Build history of the part. All positions in model axes, mm. A direction names the side the tool comes from. Coordinates: 2 decimals unless noted, no trailing zeros. Order: outer loops, then holes, each group sorted by start corner. A loop starts at its lowest first (then second) coordinate and runs counter-clockwise, first axis right, second up. Notation, with made-up numbers: (-19, 59) - (-13, 59) arc R20 ccw to (-13, 84) - close; hole circle Ø7 at (44.25, 82.25). An arc over 180 degrees is marked (long way). Write each question's results on one line, items separated by ' | '.
Autodesk Inventor part; units mm, degrees
ref_plane "Start plane" through (0, 0, -20) normal (0, 0, 1) x (1, 0, 0)
ref_plane "End plane" through (0, 0, 520) normal (0, 0, 1) x (1, 0, 0)
ref_plane "Work Plane4" through (20, 0, 520) normal (-0.7071, 0, 0.7071) x (0.7071, 0, 0.7071)
ref_plane "Start plane" through (0, 0, -20) normal (0, 0, 1) x (1, 0, 0)
ref_plane "End plane" through (0, 0, 520) normal (0, 0, 1) x (1, 0, 0)
sketch "Sketch" plane through (0, 0, 0) normal (0, 0, 1) x (1, 0, 0)
  line L0 (-20, -16.1) -> (-20, 16.1)
  line L1 (-16.1, 20) -> (16.1, 20)
  line L2 (20, 16.1) -> (20, -16.1)
  line L3 (16.1, -20) -> (-16.1, -20)
  arc A0 (-20, -16.1) -> (-16.1, -20) centre (-16.1, -16.1) ccw
  arc A1 (-16.1, 20) -> (-20, 16.1) centre (-16.1, 16.1) ccw
  arc A2 (20, 16.1) -> (16.1, 20) centre (16.1, 16.1) ccw
  arc A3 (16.1, -20) -> (20, -16.1) centre (16.1, -16.1) ccw
  line L4 (-14.8, 17.4) -> (14.8, 17.4)
  line L5 (17.4, 14.8) -> (17.4, -14.8)
  line L6 (14.8, -17.4) -> (-14.8, -17.4)
  line L7 (-17.4, -14.8) -> (-17.4, 14.8)
  line L8 (0, 29.1308) -> (0, -29.1308) construction
  line L9 (-29.1308, 0) -> (29.1308, 0) construction
  arc A4 (-17.4, -14.8) -> (-14.8, -17.4) centre (-14.8, -14.8) ccw
  arc A5 (-14.8, 17.4) -> (-17.4, 14.8) centre (-14.8, 14.8) ccw
  arc A6 (17.4, 14.8) -> (14.8, 17.4) centre (14.8, 14.8) ccw
  arc A7 (14.8, -17.4) -> (17.4, -14.8) centre (14.8, -14.8) ccw
  dimension "d7" = 3.9
  dimension "d10" = 40
  dimension "d11" = 40
  dimension "d12" = 2.6
  dimension "d15" = 20
  dimension "d16" = 20
  dimension "d19" = 2.6
  dimension "d20" = 2.6
extrude "Body" add sketch "Sketch" along normal up to surface (540 mm away) from surface at -20
sketch "Sketch3" plane through (0, 0, 0) normal (0, 0, 1) x (1, 0, 0)
  line L0 (0, 0) -> (10, 0)
ref_plane "Work Plane3" through (0, 0, 0) normal (0, -1, 0) x (1, 0, 0)
sketch "Sketch4" plane through (0, 0, 0) normal (0, -1, 0) x (1, 0, 0)
  line L0 (-2, -20) -> (12, -20)
  line L1 (-2, 520) -> (12, 520)
  dimension "d18" = 540
ref_plane "Work Plane4" through (20, 0, 520) normal (-0.7071, 0, 0.7071) x (0.7071, 0, 0.7071)
split "Split1" plane through (20, 0, 520) removes the side toward (-0.7071, 0, 0.7071)
ref_plane "Work Plane5" through (20, 0, -20) normal (-0.7071, 0, -0.7071) x (-0.7071, 0, 0.7071)
split "Split2" plane through (20, 0, -20) removes the side toward (-0.7071, 0, -0.7071)
equation "\"d7\" = G_IR"
equation "\"d10\" = G_H"
equation "\"d11\" = G_W"
equation "\"d12\" = G_T"
equation "\"d15\" = 0.5 * d10"
equation "\"d16\" = 0.5 * d11"
equation "\"d19\" = G_T"
equation "\"d20\" = G_T"
equation "\"d3\" = G_L"
equation "\"G_W\" = 40"
equation "\"G_H\" = 40"
equation "\"G_T\" = 2.6"
equation "\"G_IR\" = 3.9"
equation "\"G_L\" = d18"
properties part number "EN 10210-2 - 40 x 40 x 2.6 - 540" material "Steel, Galvanized"
1. Band-saw the part on C-C on z = 337.5. Give the cut face in (x, y).
Solved:
outline: (-20, -16.1) arc R3.9 ccw to (-16.1, -20) - (16.1, -20) arc R3.9 ccw to (20, -16.1) - (20, 16.1) arc R3.9 ccw to (16.1, 20) - (-16.1, 20) arc R3.9 ccw to (-20, 16.1) - close; hole (-17.4, -14.8) arc R2.6 ccw to (-14.8, -17.4) - (14.8, -17.4) arc R2.6 ccw to (17.4, -14.8) - (17.4, 14.8) arc R2.6 ccw to (14.8, 17.4) - (-14.8, 17.4) arc R2.6 ccw to (-17.4, 14.8) - close
2. Band-saw the part on B-B on x = -4.5. Give the cut face in (y, z).
Solved:
outline: (-20, 4.5) - (-17.4, 4.5) - (-17.4, 495.5) - (-20, 495.5) - close; (17.4, 4.5) - (20, 4.5) - (20, 495.5) - (17.4, 495.5) - close
3. Drop a flat-ended pin along its axis: pin 1 Ø5 at (x, y) = (14.5, 8) entering from +Z. Give the stop position or say it passes through.
Solved:
pin 1: passes through
4. Probe line 1 (Y direction, x = -10.5, z = 52); line 2 (X direction, y = -15.5, z = 219.5). List the from-to ranges inside material, lowest first.
Solved:
line 1: y = -20 to -17.4, 17.4 to 20 | line 2: x = -20 to -17.3, 17.3 to 20
5. Two-plate mould, pull along X, no slides. Class faces 3 (the face through (-20, 0, 247)), 4 (the face through (0, 17.4, 246)), 5 (the face through (0, 20, 246)): +X half, -X half, draft (parallel to the pull), parting line (faces both ways), or undercut.
Solved:
face 3: -X half | face 4: undercut | face 5: draft
6. Band-saw the part on A-A on y = -5.5. Give the cut face in (x, z), then the cut area to 3 significant figures.
Solved:
outline: (-20, 20) - (-17.4, 17.4) - (-17.4, 482.6) - (-20, 480) - close; (17.4, -17.4) - (20, -20) - (20, 520) - (17.4, 517.4) - close | area: 2,600 mm2
7. Tool access for faces 1 (the face through (0, -18, 500)), 2 (the face through (17.4, 0, 246)): list every direction of +Z, -Z, +X, -X, +Y, -Y with a clear straight run to the whole face (end or side of a thin tool).
Solved:
face 1: +Z, -X, +Y, -Y | face 2: +Z, -Z
